Design review of the part built by this model. Coordinates are the model's own, in mm. A direction names the side the tool comes from. Coordinates: 2 decimals unless noted, no trailing zeros. Write each loop counter-clockwise with the first axis right and the second up, starting at its lowest first coordinate (ties: lowest second). Pieces come first, ordered by that corner, then holes. Notation, with made-up numbers: (43, 76.5) - (57, 76.5) arc R22 cw to (57, 107.5) - close; hole circle Ø2 at (-32.5, 15.25). An arc over 180 degrees is marked (long way). Answer as a JSON object with one key per item and string values.
```python
from build123d import *

# Parameters (mm, degrees)
SKETCH1_W           = 44
SKETCH1_H           = 5
BOSS_EXTRUDE1_DEPTH = 32
SKETCH2_R           = 2.75
CUT_EXTRUDE1_DEPTH  = 6
BOSS_EXTRUDE2_DEPTH = 5
FILLET1_R           = 6


with BuildPart() as part:
    # Sketch1 → Boss-Extrude1 (new body)
    with BuildSketch(Plane.XY):
        with Locations((22, -2.5)):
            Rectangle(SKETCH1_W, SKETCH1_H)
    extrude(amount=BOSS_EXTRUDE1_DEPTH)

    # Sketch2 → Cut-Extrude1 (cut, through all)
    with BuildSketch(Plane.XZ.offset(5)):
        with Locations((10, 26)):
            Circle(SKETCH2_R)
        with Locations((10, 6)):
            Circle(SKETCH2_R)
        with BuildLine():
            Line((29.45, 5.75), (29.45, 4.25))
            Line((29.45, 4.25), (34.55, 4.25))
            Line((34.55, 4.25), (34.55, 5.75))
            add(Edge.make_bspline(
                [(34.55, 5.75), (50.535539216, 16), (34.55, 26.25)],
                knots=[3.521580401, 3.521580401, 3.521580401, 5.90319756, 5.90319756, 5.90319756], degree=2, weights=[1, 0.370909091, 1]))
            Line((34.55, 26.25), (34.55, 27.75))
            Line((34.55, 27.75), (29.45, 27.75))
            Line((29.45, 27.75), (29.45, 26.25))
            add(Edge.make_bspline(
                [(29.45, 26.25), (13.464460784, 16), (29.45, 5.75)],
                knots=[0.379987747, 0.379987747, 0.379987747, 2.761604906, 2.761604906, 2.761604906], degree=2, weights=[1, 0.370909091, 1]))
        make_face()
    extrude(amount=-CUT_EXTRUDE1_DEPTH, mode=Mode.SUBTRACT)

    # Sketch3 → Boss-Extrude2 (add)
    with BuildSketch(Plane.XZ.offset(5)):
        with BuildLine():
            Line((44, 32), (44, 0))
            ThreePointArc((44, 0), (48.622844919, 16), (44, 32))
        make_face()
    extrude(amount=-BOSS_EXTRUDE2_DEPTH)

    # Fillet1
    fillet1_edges = [part.edges().sort_by_distance(p)[0] for p in [
        (0, -2.5, 32),
        (44, -2.5, 32),
        (0, -2.5, 0),
        (44, -2.5, 0),
    ]]
    fillet(fillet1_edges, radius=FILLET1_R)


solid = part.part
```
(1) For pin 1 (7 mm diameter, centred on x = 10, z = 26, fed in from +Y); pin 2 (1.2 mm diameter, centred on y = -3.5, z = 4.5, fed in from -X), all flat-tipped, find the tip position at first contact; note any pin that passes through.
Solved:
{"pin 1": "stops at y = 0", "pin 2": "stops at x = 0.07"}
(2) The part is to be moulded in two halves that separate along X. For faces 3 (the face through (9.642, -2.535, 28.727)), 4 (the face through (23, -2, 0)), 5 (the face through (43.721, -2.465, 31.024)), 6 (the face through (32, -3, 4.25)), say which applies: pulls with the +X half, pulls with the -X half, needs draft (parallel to the pull), parting line crosses it, or undercut.
Solved:
{"face 3": "undercut", "face 4": "needs draft", "face 5": "pulls with the +X half", "face 6": "undercut"}
(3) Take a section at B-B, the plane y = -0.7. Give the number of separate pieces and of enclosed holes in the cut face, and give its area (3 significant figures).
Solved:
{"separate pieces": "1", "enclosed holes": "3", "area": "1,190 mm^2"}
(4) Tool access review of faces 1 (the face through (34.55, -3, 5)), 2 (the face through (48.622, -2.535, 15.819)): name each direction out of +Z, -Z, +X, -X, +Y, -Y from which nothing blocks a thin tool from reaching the whole face with its end or side.
Solved:
{"face 1": "+Y, -Y", "face 2": "+X, +Y, -Y"}
(5) To check wall thickness, follow line 1 (Z direction, x = 10, y = -3); line 2 (Z direction, x = 31.5, y = -2.4); line 3 (Z direction, x = 8.5, y = -4.7). State the ranges of each line that lie inside material, in increasing order. Write a range as from..to.
Solved:
{"line 1": "z = 0..3.25, 8.75..23.25, 28.75..32", "line 2": "z = 0..4.25, 27.75..32", "line 3": "z = 0..3.7, 8.3..23.7, 28.3..32"}
(6) Take a section at A-A, the plane x = 10. Write out the cut boundary in (y, z), and give its area (3 significant figures).
Solved:
{"outline": "(-5, 0) - (0, 0) - (0, 3.25) - (-5, 3.25) - close; (-5, 8.75) - (0, 8.75) - (0, 23.25) - (-5, 23.25) - close; (-5, 28.75) - (0, 28.75) - (0, 32) - (-5, 32) - close", "area": "105 mm^2"}
